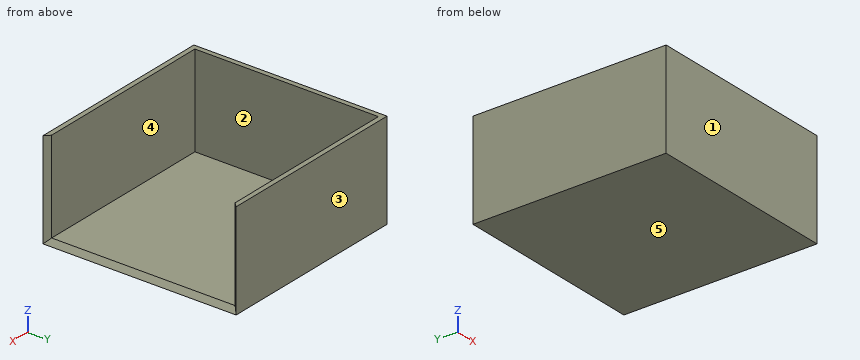
from build123d import *

# Parameters (mm, degrees)
F0_W         = 127
F0_H         = 127
F1_DEPTH     = 63.5
F2_W         = 120.65
F2_H         = 120.65
F2_W_2       = 40.16652188
F3_DEPTH     = 60.325
F4_T1_DEPTH  = 69.1433009657
F4_T3_DEPTH  = 120.65
F4_T9_DEPTH  = 129.4683009657
F4_T15_DEPTH = 69.1433009657
F4_T24_DEPTH = 69.1433009657
F4_T30_DEPTH = 129.4683009657


# Not quite as in the source:
# - a fillet or chamfer that OpenCascade refuses, or shapes differently, is made with other operations: its cross-section is extruded or revolved along the edge and cut away or added


with BuildPart() as f1:
    # F0 (on Top) → F1 (new body)
    with BuildSketch(Plane.XY):
        with Locations((9.8422262818, 3.4245376295)):
            Rectangle(F0_W, F0_H)
    extrude(amount=F1_DEPTH)

    # F2 (on face) → F3 (cut)
    with BuildSketch(Plane.XY.offset(63.5)):
        with Locations((9.8422262818, 3.4245376295)):
            Rectangle(F2_W, F2_H)
        with Locations((90.2504872218, 3.4245376295)):
            Rectangle(F2_W_2, F2_H)
    extrude(amount=-F3_DEPTH, mode=Mode.SUBTRACT)

    # F4: chamfer of 3.429 on 3 edges, made by hand

    # F4_s2 → F4_t1 (cut)
    with BuildSketch(Plane.XY.offset(3.175)):
        Polygon((73.3422262818, -60.3294623705), (69.9132262818, -56.9004623705), (73.3422262818, -56.9004623705), align=None)
        Polygon((73.3422262818, 67.1785376295), (69.9132262818, 63.7495376295), (73.3422262818, 63.7495376295), align=None)
    extrude(amount=F4_T1_DEPTH, mode=Mode.SUBTRACT)

    # F4_s4 → F4_t3 (cut)
    with BuildSketch(Plane.XZ.offset(-63.7495376295)):
        Polygon((73.3422262818, -0.254), (69.9132262818, 3.175), (73.3422262818, 3.175), align=None)
    extrude(amount=F4_T3_DEPTH, mode=Mode.SUBTRACT)


with BuildPart() as f4_tool7:
    # F4_s8 → F4_t9 (new body)
    with BuildSketch(Plane.XZ.offset(65.7187633362)):
        Polygon((73.3422262818, -0.254), (69.9132262818, 3.175), (73.3422262818, 3.175), align=None)
    extrude(amount=-F4_T9_DEPTH)

    split(bisect_by=Plane.XZ.offset(60.0754623705), keep=Keep.BOTTOM)

    split(bisect_by=Plane.XY, keep=Keep.TOP)

    split(bisect_by=Plane.XZ.offset(56.9004623705), keep=Keep.TOP)


with BuildPart() as f4_tool13:
    # F4_s14 → F4_t15 (new body)
    with BuildSketch(Plane.XY.offset(-5.6433009657)):
        Polygon((73.3422262818, -60.3294623705), (69.9132262818, -56.9004623705), (73.3422262818, -56.9004623705), align=None)
    extrude(amount=F4_T15_DEPTH)

    split(bisect_by=Plane.XZ.offset(60.0754623705), keep=Keep.BOTTOM)

    split(bisect_by=Plane.XY, keep=Keep.TOP)

    split(bisect_by=Plane.XY.offset(3.175), keep=Keep.BOTTOM)


with BuildPart() as f4_tool7_1:
    add(f4_tool7.part)

    # F4_t19: intersect F4_tool13
    add(f4_tool13.part, mode=Mode.INTERSECT)


with BuildPart() as f1_1:
    add(f1.part)

    # F4_t5: cut F4_tool7
    add(f4_tool7_1.part, mode=Mode.SUBTRACT)


with BuildPart() as f4_tool22:
    # F4_s23 → F4_t24 (new body)
    with BuildSketch(Plane.XY.offset(63.5)):
        Polygon((73.3422262818, 67.1785376295), (69.9132262818, 63.7495376295), (73.3422262818, 63.7495376295), align=None)
    extrude(amount=-F4_T24_DEPTH)

    split(bisect_by=Plane.XY, keep=Keep.TOP)

    split(bisect_by=Plane.XZ.offset(-66.9245376295), keep=Keep.TOP)

    split(bisect_by=Plane.XY.offset(3.175), keep=Keep.BOTTOM)


with BuildPart() as f4_tool28:
    # F4_s29 → F4_t30 (new body)
    with BuildSketch(Plane.XZ.offset(56.9004623705)):
        Polygon((73.3422262818, -0.254), (69.9132262818, 3.175), (73.3422262818, 3.175), align=None)
    extrude(amount=-F4_T30_DEPTH)

    split(bisect_by=Plane.XY, keep=Keep.TOP)

    split(bisect_by=Plane.XZ.offset(-66.9245376295), keep=Keep.TOP)

    split(bisect_by=Plane.XZ.offset(-63.7495376295), keep=Keep.BOTTOM)


with BuildPart() as f4_tool22_1:
    add(f4_tool22.part)

    # F4_t34: intersect F4_tool28
    add(f4_tool28.part, mode=Mode.INTERSECT)


with BuildPart() as f1_2:
    add(f1_1.part)

    # F4_t20: cut F4_tool22
    add(f4_tool22_1.part, mode=Mode.SUBTRACT)


solid = f1_2.part
Design review of the part built by this model. Coordinates are the model's own, in mm. Face numbers are marked on the shaded views. A direction names the side the tool comes from. Give positions to 0.01 mm unless a question says otherwise; leave off trailing zeros. Write each loop counter-clockwise with the first axis right and the second up, starting at its lowest first coordinate (ties: lowest second). Pieces come first, ordered by that corner, then holes. Notation, with made-up numbers: M 5,6 L 47,6 A9 ccw 47,22 Z; hole C 82,-6 d11. An arc over 180 degrees is marked long. Return JSON: item names as keys, results as strings. Group by question number.
Item 1: Clearance check with flat-ended pins moving along their axes: pin 1 Ø18 at (y, z) = (17.5, 32) entering from +X; pin 2 Ø1.5 at (x, y) = (-38.5, 50) entering from +Z (3 decimals). State where each tip first meets the part, or that it passes through.
Item 2: The part is to be moulded in two halves that separate along Y. For the marked faces 3, 4 and 5, say which applies: pulls with the +Y half, pulls with the -Y half, needs draft (parallel to the pull), parting line crosses it, or undercut.
Item 3: Wall thickness on line 1 along Y through (x, z) = (60.5, 56); line 2 along X through (y, z) = (2, 53); line 3 along Z through (x, y) = (10, 59.5) (3 decimals): over which ranges is each line inside the solid? List them lowest first.
Item 4: Take a section at A-A (x = 36). Give the boundary of the cut face in (y, z) (3 decimals), plus the area to 3 significant figures.
Item 5: Tool access review of the marked faces 1 and 2: name each direction out of +Z, -Z, +X, -X, +Y, -Y from which nothing blocks a thin tool from reaching the whole face with its end or side.
Item 6: Take a section at B-B (z = 39.5). Give the boundary of the cut face in (x, y).
Item 7: Take a section at C-C (y = -28.5). Give the boundary of the cut face in (x, z) (3 decimals).
Return value:
{
 "1": {"pin 1": "stops at x = -50.48", "pin 2": "stops at z = 3.175"},
 "2": {"face 3": "pulls with the +Y half", "face 4": "undercut", "face 5": "needs draft"},
 "3": {"line 1": "y = -60.08 to -56.9, 63.75 to 66.92", "line 2": "x = -53.66 to -50.48", "line 3": "z = 0 to 3.175"},
 "4": {"outline": "M -60.075,0 L 66.925,0 L 66.925,63.5 L 63.75,63.5 L 63.75,3.175 L -56.9,3.175 L -56.9,63.5 L -60.075,63.5 Z", "area": "786 mm2"},
 "5": {"face 1": "+Z, -Z, +X, -X, -Y", "face 2": "+Z, +X"},
 "6": {"outline": "M -53.66,-60.08 L 73.09,-60.08 L 69.91,-56.9 L -50.48,-56.9 L -50.48,63.75 L 69.91,63.75 L 73.09,66.92 L -53.66,66.92 Z"},
 "7": {"outline": "M -53.658,0 L 73.088,0 L 69.913,3.175 L -50.483,3.175 L -50.483,63.5 L -53.658,63.5 Z"}
}
